Input: part model. Units: mm. Frame: model coordinates. A direction names the side the tool comes from. Coordinates: 2 decimals unless noted, no trailing zeros. Write each loop counter-clockwise with the first axis right and the second up, starting at its lowest first coordinate (ties: lowest second). Pieces come first, ordered by that corner, then holes. Notation, with made-up numbers: M 44,-2 L 98,-2 A7 ccw 98,9 Z; hole C -18.5,25 d11. An arc over 180 degrees is marked long. Use CSV: the item, a comma, the result in double quotes.
```python
from build123d import *

# Parameters (mm, degrees)
SKETCH1_W           = 50
SKETCH1_H           = 20
BOSS_EXTRUDE1_DEPTH = 8
SKETCH2_W           = 20
SKETCH2_H           = 8
BOSS_EXTRUDE2_DEPTH = 20
RIB3_REACH          = 40.846
SKETCH3_WALL_W      = 103.015505978
SKETCH3_WALL_H      = 20
CUT_EXTRUDE3_START  = -3
SKETCH9_R           = 5
CUT_EXTRUDE3_DEPTH  = 12
SKETCH10_R          = 3
CUT_EXTRUDE4_DEPTH  = 7
RIB4_REACH          = 44.532
SKETCH12_WALL_W     = 112.064681272
SKETCH12_WALL_H     = 4.5
RIB7_REACH          = 44.532
SKETCH13_WALL_W     = 112.064681272
SKETCH13_WALL_H     = 4.5
SKETCH7_R           = 5
CUT_EXTRUDE5_DEPTH  = 1
SKETCH14_R          = 3
CUT_EXTRUDE6_DEPTH  = 7
LPATTERN1_COUNT     = 2
LPATTERN1_PITCH     = 31
SKETCH15_W          = 5.8
SKETCH15_H          = 3
BOSS_EXTRUDE3_DEPTH = 10
FILLET1_R           = 3
FILLET2_R           = 3


with BuildPart() as part:
    # Sketch1 → Boss-Extrude1 (new body)
    with BuildSketch(Plane(origin=(0, 0, 0), x_dir=(1, 0, 0), z_dir=(0, 1, 0))):
        Rectangle(SKETCH1_W, SKETCH1_H)
    extrude(amount=BOSS_EXTRUDE1_DEPTH)

    # Sketch2 → Boss-Extrude2 (add)
    with BuildSketch(Plane(origin=(0, 8, 0), x_dir=(1, 0, 0), z_dir=(0, 1, 0))):
        with Locations((0, 6)):
            Rectangle(SKETCH2_W, SKETCH2_H)
    extrude(amount=BOSS_EXTRUDE2_DEPTH)

    # Sketch3 wall → Rib3 (add, up to next)
    with BuildSketch(Plane(origin=(0, 18, 4), x_dir=(0, -0.857492925713, 0.514495755428), z_dir=(0, -0.514495755428, -0.857492925713)), mode=Mode.PRIVATE) as rib3_sk1:
        Rectangle(SKETCH3_WALL_W, SKETCH3_WALL_H)
    rib3_tool1 = extrude(rib3_sk1.sketch, amount=RIB3_REACH, mode=Mode.PRIVATE) - part.part
    add(rib3_tool1.solids().sort_by_distance((0, 18, 4))[0])

    # Sketch9 → Cut-Extrude3 (cut)
    with BuildSketch(Plane.XY.offset(CUT_EXTRUDE3_START)):
        with Locations(Location((0, 18, 0), (0, 0, 90))):
            Circle(SKETCH9_R)
    extrude(amount=CUT_EXTRUDE3_DEPTH, mode=Mode.SUBTRACT)

    # Sketch10 → Cut-Extrude4 (cut)
    with BuildSketch(Plane.XY.offset(-3)):
        with Locations((0, 18)):
            Circle(SKETCH10_R)
    extrude(amount=-CUT_EXTRUDE4_DEPTH, mode=Mode.SUBTRACT)

    # Sketch12 wall → Rib4 (add, up to next)
    with BuildSketch(Plane(origin=(-17.5, 18, -10), x_dir=(-0.6, -0.8, 0), z_dir=(-0.8, 0.6, 0)), mode=Mode.PRIVATE) as rib4_sk1:
        with Locations((0, 2.25)):
            Rectangle(SKETCH12_WALL_W, SKETCH12_WALL_H)
    rib4_tool1 = extrude(rib4_sk1.sketch, amount=-RIB4_REACH, mode=Mode.PRIVATE) - part.part
    add(rib4_tool1.solids().sort_by_distance((-17.5, 18, -10))[0])

    # Sketch13 wall → Rib7 (add, up to next)
    with BuildSketch(Plane(origin=(17.5, 18, -10), x_dir=(0.6, -0.8, 0), z_dir=(-0.8, -0.6, 0)), mode=Mode.PRIVATE) as rib7_sk1:
        with Locations((0, 2.25)):
            Rectangle(SKETCH13_WALL_W, SKETCH13_WALL_H)
    rib7_tool1 = extrude(rib7_sk1.sketch, amount=RIB7_REACH, mode=Mode.PRIVATE) - part.part
    add(rib7_tool1.solids().sort_by_distance((17.5, 18, -10))[0])

    # Sketch7 → Cut-Extrude5 (cut)
    with BuildSketch(Plane(origin=(0, 8, 0), x_dir=(1, 0, 0), z_dir=(0, 1, 0))):
        with Locations(Location((-15.5, 0, 0), (0, 0, 270))):
            Circle(SKETCH7_R)
    cut_extrude5 = extrude(amount=-CUT_EXTRUDE5_DEPTH, mode=Mode.SUBTRACT)

    # Sketch14 → Cut-Extrude6 (cut)
    with BuildSketch(Plane(origin=(0, 7, 0), x_dir=(1, 0, 0), z_dir=(0, 1, 0))):
        with Locations(Location((-15.5, 0, 0), (0, 0, 270))):
            Circle(SKETCH14_R)
    cut_extrude6 = extrude(amount=-CUT_EXTRUDE6_DEPTH, mode=Mode.SUBTRACT)

    # LPattern1: Cut-Extrude5, Cut-Extrude6 ×2
    with Locations(*[(i * LPATTERN1_PITCH, 0, 0) for i in range(1, LPATTERN1_COUNT)]):
        add(cut_extrude5, mode=Mode.SUBTRACT)
        add(cut_extrude6, mode=Mode.SUBTRACT)

    # Sketch15 → Boss-Extrude3 (add)
    with BuildSketch(Plane.XZ):
        with Locations((0, -11.5)):
            Rectangle(SKETCH15_W, SKETCH15_H)
    extrude(amount=-BOSS_EXTRUDE3_DEPTH)

    # Fillet1
    fillet1_edges = [part.edges().sort_by_distance(p)[0] for p in [
        (-25, 4, 10),
    ]]
    fillet(fillet1_edges, radius=FILLET1_R)

    # Fillet2
    fillet2_edges = [part.edges().sort_by_distance(p)[0] for p in [
        (25, 4, 10),
    ]]
    fillet(fillet2_edges, radius=FILLET2_R)


solid = part.part
```
1. Access query for faces 1 (the flat face through (15, 16, -5.5)), 2 (the cylindrical face through (10.62, 7.51, -1.08)), 3 (the flat face through (-2.9, 5, -12)), 4 (the cylindrical face through (0, 13, 1)). Directions: +Z, -Z, +X, -X, +Y, -Y. A direction counts if a zero-diameter tool reaches every point of the face in a straight line with its end or side. Return the directions, or none.
Resolved:
face 1,"+Z, +X, +Y"
face 2,"+Y"
face 3,"-Z, -X, +Y, -Y"
face 4,"+Z"
2. Section A-A (z = 0). Return loops of the section in (x, y).
Resolved:
outline,"M -25,0 L -18.5,0 L -18.5,7 L -20.5,7 L -20.5,8 L -25,8 Z; M -12.5,0 L 12.5,0 L 12.5,7 L 10.5,7 L 10.5,8 L 10,8 L 10,24.67 L -10,24.67 L -10,8 L -10.5,8 L -10.5,7 L -12.5,7 Z; M 18.5,0 L 25,0 L 25,8 L 20.5,8 L 20.5,7 L 18.5,7 Z; hole C 0,18 d10"
3. Material intervals for line 1 (X direction, y = 1.5, z = 0); line 2 (X direction, y = 7.35, z = 0); line 3 (X direction, y = 18, z = 3.75), sorted ascending. Write a range as [from, to].
Resolved:
line 1,"x = [-25, -18.5], [-12.5, 12.5], [18.5, 25]"
line 2,"x = [-25, -20.5], [-10.5, 10.5], [20.5, 25]"
line 3,"x = [-10, -5], [5, 10]"
4. Section B-B (y = 15.75). Return loops of the section in (x, z), then the cut area to 3 significant figures.
Resolved:
outline,"M -19.19,-10 L -1.98,-10 L -1.98,-3 L -4.47,-3 L -4.47,5.35 L -10,5.35 L -10,-5.5 L -19.19,-5.5 Z; M 1.98,-10 L 19.19,-10 L 19.19,-5.5 L 10,-5.5 L 10,5.35 L 4.47,5.35 L 4.47,-3 L 1.98,-3 Z"
area,"287 mm^2"
5. Mould query, pull axis Z, two halves, no side actions, for faces 5 (the cylindrical face through (-24.1, 4.06, 9.14)), 6 (the cylindrical face through (-20.38, 7.51, -1.08)), 7 (the flat face through (10, 16, -1)), 8 (the flat face through (0, 5, -13)). Classes: pulls with the +Z half, pulls with the -Z half, needs draft (parallel to the pull), parting line crosses it, or undercut.
Resolved:
face 5,"pulls with the +Z half"
face 6,"undercut"
face 7,"needs draft"
face 8,"pulls with the -Z half"
6. Contact query for flat-ended pins moving along their axis: pin 1 Ø4.5 at (y, z) = (19, 0) entering from -X; pin 2 Ø7 at (x, z) = (15.5, 0) entering from -Y; pin 3 Ø1.5 at (x, y) = (-14.5, 16) entering from -Z; pin 4 Ø6 at (y, z) = (17, -10) entering from -X. Output: stop coordinate, or through.
Resolved:
pin 1,"stops at x = -10"
pin 2,"stops at y = 0"
pin 3,"stops at z = -10"
pin 4,"stops at x = -20.5"
7. Section D-D (x = 7). Return loops of the section in (y, z).
Resolved:
outline,"M 0,-10 L 28,-10 L 28,-2 L 8,10 L 0,10 Z"
8. Section C-C (x = 15.5). Return loops of the section in (y, z), then the cut area to 3 significant figures.
Resolved:
outline,"M 0,-10 L 20.67,-10 L 20.67,-5.5 L 8,-5.5 L 8,-5 L 7,-5 L 7,-3 L 0,-3 Z; M 0,3 L 7,3 L 7,5 L 8,5 L 8,10 L 0,10 Z"
area,"165 mm^2"
